For this review, take the finished solid that the model builds, in its own axes (mm). A direction names the side the tool comes from. Give positions to 0.01 mm unless a question says otherwise; leave off trailing zeros. Loops run counter-clockwise (first coordinate to the right, second up) from the corner with the lowest first, then second, coordinate; pieces in that order, holes last. Notation, with made-up numbers: (-15.5, -26.75) -> (-5.5, -26.75) arc R13 cw to (-5.5, -16.75) -> close; hole circle Ø5 at (7.25, -7.5). An arc over 180 degrees is marked (long way). Write each question's results on one line, items separated by ' | '. Start each with the question number.
```python
from build123d import *

# Parameters (mm, degrees)
BOSS_EXTRUDE1_DEPTH      = 50
CUT_EXTRUDE1_DEPTH       = 71.328210001
CUT_EXTRUDE1_DEPTH_BACK  = 71.328210001
SKETCH3_W                = 43
SKETCH3_H                = 41.467755669
BOSS_EXTRUDE3_DEPTH      = 5
BOSS_EXTRUDE3_DEPTH_BACK = 5
CUT_EXTRUDE2_REACH       = 78.643
SKETCH6_R                = 1


with BuildPart() as part:
    # Sketch1 → Boss-Extrude1 (new body)
    with BuildSketch(Plane.XY):
        with BuildLine():
            Line((0, 34.943627773), (0, 26.943627773))
            ThreePointArc((0, 26.943627773), (-4, 22.943627773), (0, 18.943627773))
            Line((0, 18.943627773), (0, 0))
            Line((0, 0), (-35, 0))
            Line((-35, 0), (-35, 2))
            ThreePointArc((-35, 2), (-19.845914105, 8.458947707), (-12, 22.943627773))
            ThreePointArc((-12, 22.943627773), (-8.485281374, 31.428909148), (0, 34.943627773))
        make_face()
    boss_extrude1 = extrude(amount=BOSS_EXTRUDE1_DEPTH)

    # Mirror1: Boss-Extrude1 across plane
    add(boss_extrude1.mirror(Plane(origin=(0, 18.943627773, 50), x_dir=(0, 0, 1), z_dir=(-1, 0, 0))))

    # Sketch3 → Cut-Extrude1 (cut, two sides: drawn at the far end of the back side and taken through both)
    with BuildSketch(Plane(origin=(0, 0, 0), x_dir=(0, 0, -1), z_dir=(1, 0, 0)).offset(-CUT_EXTRUDE1_DEPTH_BACK)):
        with Locations((-25, 22.733877835)):
            Rectangle(SKETCH3_W, SKETCH3_H)
    extrude(amount=CUT_EXTRUDE1_DEPTH + CUT_EXTRUDE1_DEPTH_BACK, mode=Mode.SUBTRACT)

    # Sketch5 → Boss-Extrude3 (add, two sides: drawn at the far end of the back side and taken through both)
    with BuildSketch(Plane.ZY.offset(-BOSS_EXTRUDE3_DEPTH_BACK)):
        Polygon((-7.365906047, 6.54), (-7.365906047, 1.184093953), (0, 1.184093953), (0, 0), (-8.55, 0), (-8.55, 6.54), align=None)
        Polygon((0, 32.943627773), (0, 33.943627773), (-8.55, 33.943627773), (-8.55, 29.943627773), (-7.365906047, 29.943627773), (-7.365906047, 32.943627773), align=None)
    extrude(amount=BOSS_EXTRUDE3_DEPTH + BOSS_EXTRUDE3_DEPTH_BACK)

    # Sketch6 → Cut-Extrude2 (cut, up to next)
    with BuildSketch(Plane(origin=(0, 0, -8.55), x_dir=(-1, 0, 0), z_dir=(0, 0, -1)), mode=Mode.PRIVATE) as cut_extrude2_sk1:
        with Locations((0, 3.88)):
            Circle(SKETCH6_R)
    cut_extrude2_tool1 = extrude(cut_extrude2_sk1.sketch, amount=-CUT_EXTRUDE2_REACH, mode=Mode.PRIVATE) & part.part
    # Sketch6 → Cut-Extrude2 (cut, up to next)
    with BuildSketch(Plane(origin=(0, 0, -8.55), x_dir=(-1, 0, 0), z_dir=(0, 0, -1)), mode=Mode.PRIVATE) as cut_extrude2_sk2:
        with Locations((0, 31.690394603)):
            Circle(SKETCH6_R)
    cut_extrude2_tool2 = extrude(cut_extrude2_sk2.sketch, amount=-CUT_EXTRUDE2_REACH, mode=Mode.PRIVATE) & part.part
    add(cut_extrude2_tool1.solids().sort_by_distance((0, 3.88, -8.55))[0], mode=Mode.SUBTRACT)
    add(cut_extrude2_tool2.solids().sort_by_distance((0, 31.690395, -8.55))[0], mode=Mode.SUBTRACT)


solid = part.part
```
1. Wall thickness on L1, parallel to Y at x = 0, z = -7.65; L2, parallel to Y at x = 0, z = -7; L3, parallel to Z at x = 9, y = 13: over which ranges is each line inside the solid? List them lowest first.
2. We need section D-D (x = -9.5). Write out the cut boundary in (y, z).
3. Draft analysis for pull direction Z (two halves, no side actions). For faces 5 (the cylindrical face through (20.02, 8.3, 48.23)), 6 (the flat face through (0, 2, -8.55)), 7 (the flat face through (0, 32.944, -4)), state which applies: released by +Z, released by -Z, zero draft, split by the parting line, or undercut.
4. We need section B-B (x = -2). Write out the cut boundary in (y, z).
5. For pin 1 Ø10 at (x, z) = (16.5, 2) entering from -Y; pin 2 Ø10 at (x, y) = (12, 15.5) entering from -Z; pin 3 Ø6 at (x, z) = (-14, 10.5) entering from +Y; pin 4 Ø1 at (x, y) = (-19, 10.5) entering from +Z, all flat-tipped, find the tip position at first contact; note any pin that passes through.
6. We need section C-C (y = 24.5). Write out the cut boundary in (x, z).
7. We need section A-A (z = -1). Write out the cut boundary in (x, y).
8. Machinability: for faces 1 (the flat face through (0, 15, 46.5)), 2 (the flat face through (5, 1, -6)), 3 (the flat face through (-5, 1, -6)), 4 (the flat face through (0.1, 30.4, -7.366)), which of the approach directions +Z, -Z, +X, -X, +Y, -Y give a long, thin tool a straight path to every point of the face, cutting with its end or side? Answer none if there is none.
Response:
1) L1: y = 0 to 2.88, 4.88 to 6.54, 29.94 to 30.69, 32.69 to 33.94 | L2: y = 0 to 1.18, 32.94 to 33.94 | L3: z = 0 to 3.5, 46.5 to 50
2) outline: (0, 0) -> (30.28, 0) -> (30.28, 3.5) -> (2, 3.5) -> (2, 46.5) -> (30.28, 46.5) -> (30.28, 50) -> (0, 50) -> close
3) face 5: zero draft | face 6: released by -Z | face 7: undercut
4) outline: (0, -8.55) -> (6.54, -8.55) -> (6.54, -7.37) -> (1.18, -7.37) -> (1.18, 0) -> (19.48, 0) -> (19.48, 3.5) -> (2, 3.5) -> (2, 46.5) -> (19.48, 46.5) -> (19.48, 50) -> (0, 50) -> close; (26.41, 0) -> (32.94, 0) -> (32.94, -7.37) -> (29.94, -7.37) -> (29.94, -8.55) -> (33.94, -8.55) -> (33.94, 0) -> (34.78, 0) -> (34.78, 3.5) -> (26.41, 3.5) -> close; (26.41, 46.5) -> (34.78, 46.5) -> (34.78, 50) -> (26.41, 50) -> close
5) pin 1: stops at y = 0 | pin 2: stops at z = 0 | pin 3: stops at y = 2 | pin 4: passes through
6) outline: (-11.9, 0) -> (-3.68, 0) -> (-3.68, 3.5) -> (-11.9, 3.5) -> close; (-11.9, 46.5) -> (-3.68, 46.5) -> (-3.68, 50) -> (-11.9, 50) -> close; (3.68, 0) -> (11.9, 0) -> (11.9, 3.5) -> (3.68, 3.5) -> close; (3.68, 46.5) -> (11.9, 46.5) -> (11.9, 50) -> (3.68, 50) -> close
7) outline: (-5, 0) -> (5, 0) -> (5, 1.18) -> (-5, 1.18) -> close; (-5, 32.94) -> (5, 32.94) -> (5, 33.94) -> (-5, 33.94) -> close
8) face 1: +X, -X, +Y | face 2: -Z, +X, +Y, -Y | face 3: -Z, -X, +Y, -Y | face 4: +X, -X
